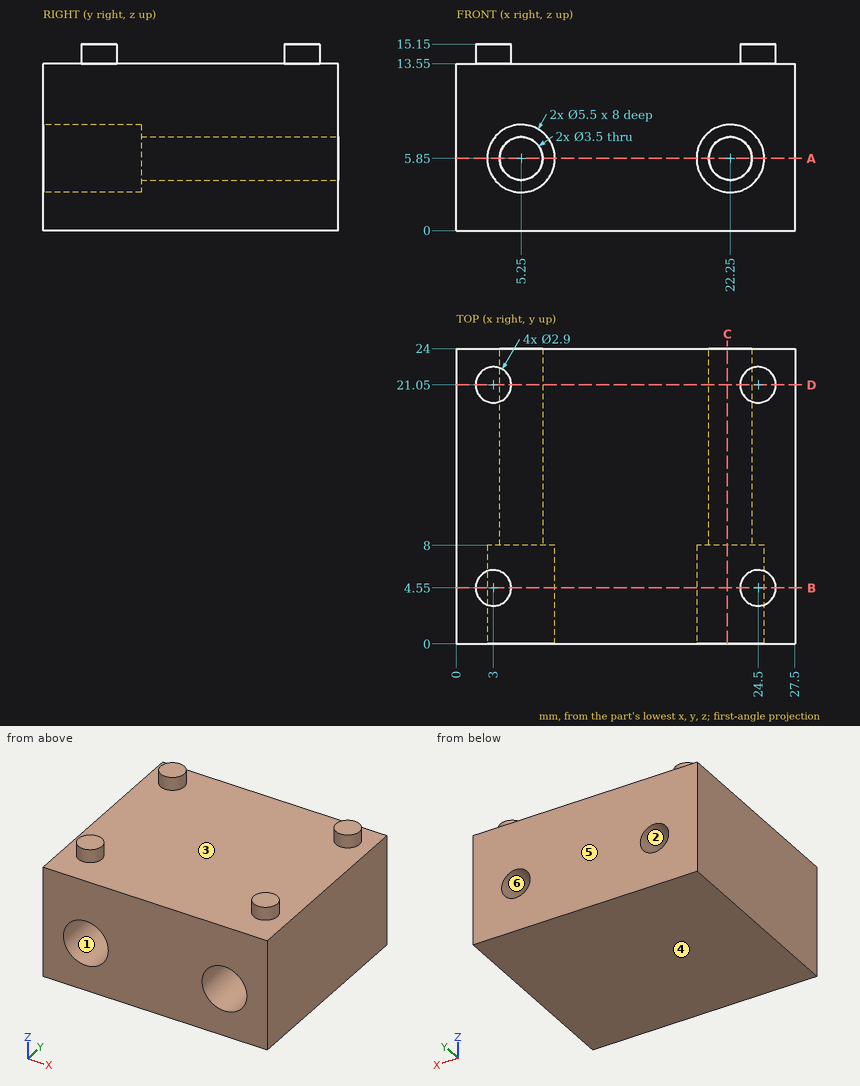
Part print with two shaded views. Sizes in mm from the minimum x, y, z corner. A direction names the side the tool comes from. Give positions to 0.01 mm unless a question says otherwise; leave off trailing zeros. Order: outer loops, then holes, each group sorted by start corner. A loop starts at its lowest first (then second) coordinate and runs counter-clockwise, first axis right, second up.
1) 3-axis set-ups, long thin cutter, end or side, ignore diameter. For the marked faces 1 and 2: which of +Z, -Z, +X, -X, +Y, -Y reach the whole face in a straight line?
2) Mould opens along Z. For the marked faces 3, 4, 5 and 6 say: +Z half, -Z half, draft (parallel to the pull), parting line (faces both ways), or undercut.
3) Saw through at C-C, the plane x = 22. Write the cut outline in (y, z), then the cut area to 3 significant figures.
4) Saw through at B-B, the plane y = 4.55. Write the cut outline in (x, z).
5) Saw through at D-D, the plane y = 21.05. Write the cut outline in (x, z).
6) Pin check, flat tips, straight feed: pin 1 (4 mm diameter, centred on x = 19.5, y = 11, fed in from +Z); pin 2 (4 mm diameter, centred on x = 22.25, z = 5.85, fed in from -Y); pin 3 (4.5 mm diameter, centred on x = 5.25, z = 5.85, fed in from +Y). Stop position of each tip, or through.
7) Wall check: probe 1 along X at (y, z) = (11.5, 5.5) (1 decimal); probe 2 along Z at (x, y) = (25.75, 10.5); probe 3 along Y at (x, z) = (23.5, 8.25). Give the ranges that are in metal, low to high.
8) Saw through at A-A, the plane z = 5.85. Write the cut outline in (x, y).
Computed:
1. face 1: -Y
1. face 2: +Y, -Y
2. face 3: +Z half
2. face 4: -Z half
2. face 5: draft
2. face 6: undercut
3. outline: (0, 0) - (24, 0) - (24, 4.12) - (8, 4.12) - (8, 3.11) - (0, 3.11) - close; (0, 8.59) - (8, 8.59) - (8, 7.58) - (24, 7.58) - (24, 13.55) - (0, 13.55) - close
3. area: 226 mm2
4. outline: (0, 0) - (27.5, 0) - (27.5, 13.55) - (25.95, 13.55) - (25.95, 15.15) - (23.05, 15.15) - (23.05, 13.55) - (4.45, 13.55) - (4.45, 15.15) - (1.55, 15.15) - (1.55, 13.55) - (0, 13.55) - close; hole circle Ø5.5 at (5.25, 5.85); hole circle Ø5.5 at (22.25, 5.85)
5. outline: (0, 0) - (27.5, 0) - (27.5, 13.55) - (25.95, 13.55) - (25.95, 15.15) - (23.05, 15.15) - (23.05, 13.55) - (4.45, 13.55) - (4.45, 15.15) - (1.55, 15.15) - (1.55, 13.55) - (0, 13.55) - close; hole circle Ø3.5 at (5.25, 5.85); hole circle Ø3.5 at (22.25, 5.85)
6. pin 1: stops at z = 13.55
6. pin 2: stops at y = 8
6. pin 3: stops at y = 24
7. probe 1: x = 0 to 3.5, 7 to 20.5, 24 to 27.5
7. probe 2: z = 0 to 13.55
7. probe 3: y = 8 to 24
8. outline: (0, 0) - (2.5, 0) - (2.5, 8) - (3.5, 8) - (3.5, 24) - (0, 24) - close; (7, 8) - (8, 8) - (8, 0) - (19.5, 0) - (19.5, 8) - (20.5, 8) - (20.5, 24) - (7, 24) - close; (24, 8) - (25, 8) - (25, 0) - (27.5, 0) - (27.5, 24) - (24, 24) - close
